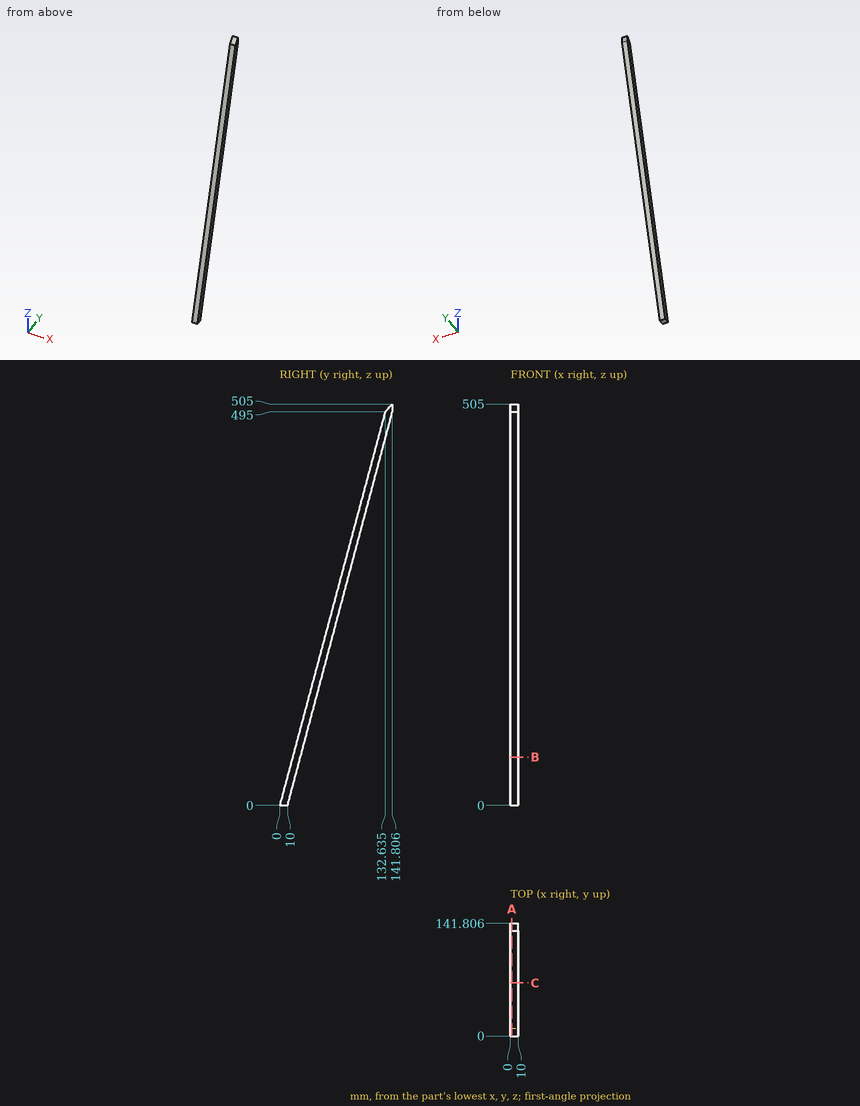
Design review of the part shown in the three views and the two pictorial views. Dimensions are in mm from the part's minimum x, y and z. Round coordinates to 2 decimals unless told otherwise and drop trailing zeros. Loops run counter-clockwise (first coordinate to the right, second up) from the corner with the lowest first, then second, coordinate; pieces in that order, holes last. Notation, with made-up numbers: (46.25, 67.5) - (77.25, 67.5) arc R21 cw to (77.25, 87.5) - close; hole circle Ø11 at (31, 81.5). An arc over 180 degrees is marked (long way). Use one line per item in the form item = value.
1) Wall thickness on probe 1 along Y at (x, z) = (6.5, 187); probe 2 along Y at (x, z) = (3, 231.5): over which ranges is each line inside the solid? List them lowest first.
Solutions:
probe_1 = 50.11 to 59.79
probe_2 = 62.03 to 71.64
2) Clearance check with flat-ended pins moving along their axes: P1, Ø6, axis at x = 5.5, z = 263.5, coming from the -Y side; P2, Ø3, axis at x = 2.5, z = 261.5, coming from the +Y side; P3, Ø3, axis at x = 4, z = 303.5, coming from the +Y side. State where each tip first meets the part, or that it passes through.
Solutions:
P1 = 69.8
P2 = 80.03
P3 = 91.21
3) We need section B-B on z = 60.5. Write out the cut boundary in (x, y).
Solutions:
outline = (0, 16.21) - (10, 16.21) - (10, 26.11) - (0, 26.11) - close
4) We need section A-A on x = 2. Write out the cut boundary in (y, z) (3 decimals).
Solutions:
outline = (0, 0) - (10, 0) - (141.806, 495) - (141.806, 505) - (132.635, 495) - close
5) We need section C-C on y = 67. Write out the cut boundary in (x, z).
Solutions:
outline = (0, 214.06) - (10, 214.06) - (10, 250.05) - (0, 250.05) - close
